```python
from build123d import *

# Parameters (mm, degrees)
F0_W     = 10
F0_H     = 5
F0_R     = 3
F1_DEPTH = 5


with BuildPart() as f1:
    # F0 (on Top) → F1 (new body)
    with BuildSketch(Plane.XY):
        with BuildLine():
            Line((-50, -5), (50, -5))
            Line((50, -5), (50, 0))
            ThreePointArc((50, 0), (48.535534, 3.535534), (45, 5))
            Line((45, 5), (-50, 5))
            Line((-50, 5), (-50, -5))
        make_face()
        with Locations((-30, 0)):
            Rectangle(F0_W, F0_H, mode=Mode.SUBTRACT)
        Circle(F0_R, mode=Mode.SUBTRACT)
        with BuildLine():
            ThreePointArc((35, -1), (34.56066, -2.06066), (33.5, -2.5))
            Line((33.5, -2.5), (26.5, -2.5))
            ThreePointArc((26.5, -2.5), (25.43934, -2.06066), (25, -1))
            Line((25, -1), (25, 1))
            ThreePointArc((25, 1), (25.43934, 2.06066), (26.5, 2.5))
            Line((26.5, 2.5), (33.5, 2.5))
            ThreePointArc((33.5, 2.5), (34.56066, 2.06066), (35, 1))
            Line((35, 1), (35, -1))
        make_face(mode=Mode.SUBTRACT)
    extrude(amount=F1_DEPTH)


solid = f1.part
```
Verification items for the finished model (mm, model axes). A direction names the side the tool comes from. Coordinates: 2 decimals unless noted, no trailing zeros. Order: outer loops, then holes, each group sorted by start corner. A loop starts at its lowest first (then second) coordinate and runs counter-clockwise, first axis right, second up. Notation, with made-up numbers: (46.25, 71) - (98.25, 71) arc R21 ccw to (98.25, 100) - close; hole circle Ø2 at (-34.5, -25). An arc over 180 degrees is marked (long way). Return JSON: item names as keys, results as strings.
(1) Mould release check, pull along X, two halves, no side actions. Record for faces 3 (the cylindrical face through (49, 3, 2)), 4 (the flat face through (-35, 0, 2)), 5 (the flat face through (-1, 3, 5)): pulls with the +X half, pulls with the -X half, needs draft (parallel to the pull), parting line crosses it, or undercut.
Filled sheet:
{"face 3": "pulls with the +X half", "face 4": "undercut", "face 5": "needs draft"}
(2) Thickness scan on line 1 along X through (y, z) = (-2, 3.05); line 2 along Y through (x, z) = (0, 1.9); line 3 along X through (y, z) = (2, 4.2). Record the ranges inside material, lowest first.
Filled sheet:
{"line 1": "x = -50 to -35, -25 to -2.24, 2.24 to 25.38, 34.62 to 50", "line 2": "y = -5 to -3, 3 to 5", "line 3": "x = -50 to -35, -25 to -2.24, 2.24 to 25.38, 34.62 to 49.58"}
(3) Section check A-A, the plane x = -27.5. Record the cut outline in (y, z).
Filled sheet:
{"outline": "(-5, 0) - (-2.5, 0) - (-2.5, 5) - (-5, 5) - close; (2.5, 0) - (5, 0) - (5, 5) - (2.5, 5) - close"}
(4) Access from +Z, -Z, +X, -X, +Y, -Y to the whole of each face (thin tool, end or side, straight path). Record for faces 1 (the flat face through (-1, -5, 2)), 2 (the flat face through (30, 2.5, 2)).
Filled sheet:
{"face 1": "+Z, -Z, +X, -X, -Y", "face 2": "+Z, -Z"}
(5) Section check B-B, the plane x = 0. Record the cut outline in (y, z), and give its area (3 significant figures).
Filled sheet:
{"outline": "(-5, 0) - (-3, 0) - (-3, 5) - (-5, 5) - close; (3, 0) - (5, 0) - (5, 5) - (3, 5) - close", "area": "20.0 mm^2"}
